Here's how the part is built. I have some questions about the finished solid (model axes, mm). A direction names the side the tool comes from. Round coordinates to 2 decimals unless told otherwise and drop trailing zeros. Order: outer loops, then holes, each group sorted by start corner. A loop starts at its lowest first (then second) coordinate and runs counter-clockwise, first axis right, second up. Notation, with made-up numbers: (51.25, -10) - (75.25, -10) arc R31 ccw to (75.25, 24) - close; hole circle Ø5 at (-24, -27.75). An arc over 180 degrees is marked (long way). Answer as a JSON object with one key per item and string values.
```python
from build123d import *

# Parameters (mm, degrees)
SKETCH1_R                       = 1.5
SKETCH1_R_2                     = 5.100618704
BOSS_EXTRUDE1_DEPTH             = 23
FILLET2_R                       = 50.8
SKETCH2_R                       = 40.05
CUT_EXTRUDE1_DEPTH              = 16
SKETCH5_R                       = 36.83
CUT_EXTRUDE2_DEPTH              = 25.4
FILLET5_R                       = 1
FILLET6_R                       = 1
M10_CLEARANCE_HOLE4_D           = 10.5
M10_CLEARANCE_HOLE4_CSINK_D     = 11.55
M10_CLEARANCE_HOLE4_CSINK_ANGLE = 90


with BuildPart() as part:
    # Sketch1 → Boss-Extrude1 (new body)
    with BuildSketch(Plane.XY):
        with BuildLine():
            Line((75.260281277, -167.806485638), (-4.700564051, -136.778396463))
            Line((-4.700564051, -136.778396463), (-76.156211748, -158.845068243))
            ThreePointArc((-76.156211748, -158.845068243), (-84.397046653, -158.966738807), (-91.402736844, -154.625486844))
            Line((-91.402736844, -154.625486844), (-132.961820606, -108.305285312))
            ThreePointArc((-132.961820606, -108.305285312), (-135.879409932, -103.381593327), (-136.690789762, -97.716195457))
            Line((-136.690789762, -97.716195457), (-124.255747511, 131.9473438))
            ThreePointArc((-124.255747511, 131.9473438), (-118.813814635, 142.502935513), (-107.309980144, 145.451993305))
            Line((-107.309980144, 145.451993305), (-13.820265411, 129.310675557))
            Line((-13.820265411, 129.310675557), (57.154321142, 144.67282316))
            ThreePointArc((57.154321142, 144.67282316), (66.292090414, 143.669172059), (72.989999045, 137.372810987))
            Line((72.989999045, 137.372810987), (111.561324809, 65.705034096))
            ThreePointArc((111.561324809, 65.705034096), (120.450704592, 47.507478462), (126.394675624, 28.146659461))
            Line((126.394675624, 28.146659461), (143.447960396, -48.284765241))
            ThreePointArc((143.447960396, -48.284765241), (142.753389973, -56.92050988), (137.306991007, -63.658109738))
            Line((137.306991007, -63.658109738), (104.679233021, -85.560920301))
            Line((104.679233021, -85.560920301), (95.102188007, -156.104602115))
            ThreePointArc((95.102188007, -156.104602115), (88.018421694, -166.766325043), (75.260281277, -167.806485638))
        make_face()
        with Locations((-109.776955272, 131.163395273)):
            Circle(SKETCH1_R, mode=Mode.SUBTRACT)
        with Locations((-70.826725389, 107.740981135)):
            Circle(SKETCH1_R_2, mode=Mode.SUBTRACT)
        with Locations((-122.043542394, -98.509264921)):
            Circle(SKETCH1_R, mode=Mode.SUBTRACT)
        with Locations((-80.484458632, -144.829466453)):
            Circle(SKETCH1_R, mode=Mode.SUBTRACT)
        with Locations((52.801836898, -118.009411705)):
            Circle(SKETCH1_R_2, mode=Mode.SUBTRACT)
        with Locations((80.566824551, -154.131274008)):
            Circle(SKETCH1_R, mode=Mode.SUBTRACT)
        with Locations((129.131286757, -51.479083724)):
            Circle(SKETCH1_R, mode=Mode.SUBTRACT)
        with Locations((60.221754192, 130.500990023)):
            Circle(SKETCH1_R, mode=Mode.SUBTRACT)
    extrude(amount=BOSS_EXTRUDE1_DEPTH)

    # Fillet2
    fillet2_edges = [part.edges().sort_by_distance(p)[0] for p in [
        (104.679233021, -85.560920301, 11.5),
        (-4.700564051, -136.778396463, 11.5),
        (-13.820265411, 129.310675557, 11.5),
    ]]
    fillet(fillet2_edges, radius=FILLET2_R)

    # Sketch2 → Cut-Extrude1 (cut)
    with BuildSketch(Plane(origin=(0, 0, 23), x_dir=(-1, 0, 0), z_dir=(0, 0, -1))):
        Circle(SKETCH2_R)
    extrude(amount=CUT_EXTRUDE1_DEPTH, mode=Mode.SUBTRACT)

    # Sketch5 → Cut-Extrude2 (cut)
    with BuildSketch(Plane(origin=(0, 0, 23), x_dir=(-1, 0, 0), z_dir=(0, 0, -1))):
        with Locations(Location((0, 0, 0), (0, 0, 180))):
            Circle(SKETCH5_R)
    extrude(amount=CUT_EXTRUDE2_DEPTH, mode=Mode.SUBTRACT)

    # Fillet5
    fillet5_edges = [part.edges().sort_by_distance(p)[0] for p in [
        (40.05, 0, 23),
    ]]
    fillet(fillet5_edges, radius=FILLET5_R)

    # Fillet6
    fillet6_edges = [part.edges().sort_by_distance(p)[0] for p in [
        (40.05, 0, 7),
    ]]
    fillet(fillet6_edges, radius=FILLET6_R)

    # M10 Clearance Hole4 (through all)
    with Locations(Plane.XY.offset(23)):
        with Locations((60.221754192, 130.500990023), (-109.776955272, 131.163395273), (129.131286757, -51.479083724), (80.566824551, -154.131274008), (-80.484458632, -144.829466453), (-122.043542394, -98.509264921)):
            CounterSinkHole(M10_CLEARANCE_HOLE4_D / 2, M10_CLEARANCE_HOLE4_CSINK_D / 2, counter_sink_angle=M10_CLEARANCE_HOLE4_CSINK_ANGLE)


solid = part.part
```
1. For faces 4 (the face through (43.96, -155.66, 11.34)), 5 (the face through (23, -29, 7)), 6 (the face through (26.065, 137.944, 11.339)), 7 (the face through (-85.49, -143.25, 11.08)), which set-ups out of +Z, -Z, +X, -X, +Y, -Y let a thin tool reach every point of the face, with its end or its side?
Responses:
{"face 4": "+Z, -Z, -Y", "face 5": "+Z", "face 6": "+Z, -Z, +Y", "face 7": "+Z, -Z"}
2. For P1, Ø5, axis at x = -26.5, z = 7.5, coming from the +Y side; P2, Ø9.5, axis at x = 129.13, y = -51.48, coming from the -Z side; P3, Ø8, axis at y = -76, z = 17.5, coming from the -X side; P4, Ø5, axis at x = 24, z = 2.5, coming from the -Y side, each with a flat end and sliding along its axis, tell me the tip position at first contact or that it passes through.
Responses:
{"P1": "y = 131.93", "P2": "through", "P3": "x = -135.73", "P4": "y = -148.89"}
3. Imagine slicing it at B-B (x = 0). List the corners of the cut face in (y, z) for me.
Responses:
{"outline": "(-140.16, 0) - (-36.83, 0) - (-36.83, 7) - (-39.05, 7) arc R1 cw to (-40.05, 8) - (-40.05, 22) arc R1 ccw to (-41.05, 23) - (-140.16, 23) - close; (36.83, 0) - (132.3, 0) - (132.3, 23) - (41.05, 23) arc R1 ccw to (40.05, 22) - (40.05, 8) arc R1 cw to (39.05, 7) - (36.83, 7) - close"}
4. Thinking about a two-plate mould opening in X: for faces 1 (the face through (-130.56, 15.51, 11.34)), 2 (the face through (134.8, -9.53, 11.34)), 3 (the face through (-68.5, 103.2, 11.3)), which applies, pulls with the +X half, pulls with the -X half, needs draft (parallel to the pull), parting line crosses it, or undercut?
Responses:
{"face 1": "pulls with the -X half", "face 2": "pulls with the +X half", "face 3": "undercut"}
5. Imagine slicing it at D-D (x = -50.5). List the corners of the cut face in (y, z) for me, plus the area to 3 significant figures.
Responses:
{"outline": "(-150.92, 0) - (135.64, 0) - (135.64, 23) - (-150.92, 23) - close", "area": "6,590 mm2"}
6. Imagine slicing it at A-A (y = 0). List the corners of the cut face in (x, z) for me.
Responses:
{"outline": "(-131.4, 0) - (-36.83, 0) - (-36.83, 7) - (-39.05, 7) arc R1 cw to (-40.05, 8) - (-40.05, 22) arc R1 ccw to (-41.05, 23) - (-131.4, 23) - close; (36.83, 0) - (132.67, 0) - (132.67, 23) - (41.05, 23) arc R1 ccw to (40.05, 22) - (40.05, 8) arc R1 cw to (39.05, 7) - (36.83, 7) - close"}
7. Imagine slicing it at C-C (z = 15.5). Give the number of separate pieces and of enclosed holes in the cut face, plus the area to 3 significant figures.
Responses:
{"separate pieces": "1", "enclosed holes": "9", "area": "64,600 mm2"}
8. If I drill on L1, parallel to Y at x = -120, z = 10.75; L2, parallel to X at y = -17, z = 18.5; L3, parallel to Y at x = 22.5, z = 15.5, over which ranges is the centre line in solid material (lowest first)? Write a range as [from, to].
Responses:
{"L1": "[-122.75, -103.35], [-93.67, 141.45]", "L2": "[-132.32, -36.26], [36.26, 136.47]", "L3": "[-147.33, -33.13], [33.13, 137.17]"}
